from build123d import *

# Parameters (mm, degrees)
SKETCH_1_R       = 2.45
EXTRUDE_2_DEPTH  = 2
SKETCH_1_5_R     = 2.45
EXTRUDE_3_DEPTH  = 2
SKETCH_8_R       = 2.45
EXTRUDE_5_DEPTH  = 3
SKETCH_10_R      = 2.529452546
EXTRUDE_6_DEPTH  = 2
SKETCH_11_W      = 2.5
SKETCH_11_H      = 4.5
EXTRUDE_7_DEPTH  = 2
SKETCH_1_7_W     = 10
SKETCH_1_7_H     = 1
EXTRUDE_8_DEPTH  = 23
SKETCH_13_W      = 10
SKETCH_13_H      = 1
EXTRUDE_9_DEPTH  = 2
SKETCH_21_R      = 2.45
EXTRUDE_10_DEPTH = 5


with BuildPart() as part:
    # Sketch 1 → Extrude 2 (new body)
    with BuildSketch(Plane.XY):
        with BuildLine():
            Line((-52.360741066, -3.31033927), (-60.460741066, -3.31033927))
            Line((-60.460741066, -3.31033927), (-60.460741066, -7.81033927))
            Line((-60.460741066, -7.81033927), (-56.860741066, -7.81033927))
            ThreePointArc((-56.860741066, -7.81033927), (-49.178760551, -10.992319786), (-52.360741066, -3.31033927))
        make_face()
        with Locations((-52.360741066, -7.81033927)):
            Circle(SKETCH_1_R, mode=Mode.SUBTRACT)
    extrude(amount=-EXTRUDE_2_DEPTH)



with BuildPart() as body_2:
    # Sketch 1_5 → Extrude 3 (new body)
    with BuildSketch(Plane.XY):
        with BuildLine():
            Line((-78.460741066, -12.31033927), (-70.458584645, -12.31033927))
            Line((-70.458584645, -12.31033927), (-70.458584645, -13.81033927))
            Line((-70.458584645, -13.81033927), (-60.458584645, -13.81033927))
            Line((-60.458584645, -13.81033927), (-60.460741066, -12.31033927))
            Line((-60.460741066, -12.31033927), (-60.460741066, -7.81033927))
            Line((-60.460741066, -7.81033927), (-60.460741066, -3.31033927))
            Line((-60.460741066, -3.31033927), (-78.460741066, -3.31033927))
            ThreePointArc((-78.460741066, -3.31033927), (-82.960741066, -7.81033927), (-78.460741066, -12.31033927))
        make_face()
        with Locations((-78.460741066, -7.81033927)):
            Circle(SKETCH_1_5_R, mode=Mode.SUBTRACT)
    extrude(amount=EXTRUDE_3_DEPTH)


with BuildPart() as body_3:
    # Sketch 8 → Extrude 5 (new body)
    with BuildSketch(Plane.XY):
        with Locations((-52.360741066, -7.81033927)):
            Circle(SKETCH_8_R)
    extrude(amount=EXTRUDE_5_DEPTH)


with BuildPart() as part_1:
    add(part.part)

    add(body_3.part)  # Extrude 6 merges body 3
    # Sketch 10 → Extrude 6 (add)
    with BuildSketch(Plane.XY):
        with Locations((-52.43882399, -7.795650359)):
            Circle(SKETCH_10_R)
    extrude(amount=-EXTRUDE_6_DEPTH)


    add(body_2.part)  # Extrude 7 merges body 2
    # Sketch 11 → Extrude 7 (add)
    with BuildSketch(Plane(origin=(0, 0, 0), x_dir=(-1, 0, 0), z_dir=(0, 0, -1))):
        with Locations((61.710741066, -5.56033927)):
            Rectangle(SKETCH_11_W, SKETCH_11_H)
    extrude(amount=EXTRUDE_7_DEPTH)



with BuildPart() as body_2_2:
    # Sketch 1_7 → Extrude 8 (new body)
    with BuildSketch(Plane.XY):
        with Locations((-65.458584645, -14.31033927)):
            Rectangle(SKETCH_1_7_W, SKETCH_1_7_H)
    extrude(amount=-EXTRUDE_8_DEPTH)


with BuildPart() as part_2:
    add(part_1.part)

    add(body_2_2.part)  # Extrude 9 merges body 2 2
    # Sketch 13 → Extrude 9 (add)
    with BuildSketch(Plane.XY):
        with Locations((-65.458584645, -14.31033927)):
            Rectangle(SKETCH_13_W, SKETCH_13_H)
    extrude(amount=EXTRUDE_9_DEPTH)

    # Sketch 21 → Extrude 10 (add)
    with BuildSketch(Plane(origin=(0, 0, 0), x_dir=(-1, 0, 0), z_dir=(0, 0, -1))):
        with Locations((78.465233983, -7.801636169)):
            Circle(SKETCH_21_R)
    extrude(amount=-EXTRUDE_10_DEPTH)


solid = part_2.part
Geometry: final body of the model. Coordinates: model frame, mm. A direction names the side the tool comes from. Round coordinates to 2 decimals unless told otherwise and drop trailing zeros. Loops run counter-clockwise (first coordinate to the right, second up) from the corner with the lowest first, then second, coordinate; pieces in that order, holes last.
Q1. Section D-D on x = -51. Return loops of the section in (y, z), plus the area to 3 significant figures.
Q2. Section A-A on y = -8.25. Return loops of the section in (x, z), plus the area to 3 significant figures.
Q3. Pin query (flat end, axial travel): P1, Ø12, axis at x = -55, z = -7, coming from the +Y side; P2, Ø1, axis at x = -74, z = 1, coming from the -Y side; P3, Ø2.5, axis at x = -52, y = -6.5, coming from the +Z side; P4, Ø0.8, axis at y = -14, z = -10.5, coming from the -X side. Return the tip coordinate at first contact, or that it passes through.
Q4. Material intervals for L1, parallel to Z at x = -70, y = -14; L2, parallel to Y at x = -69.5, z = -2.25; L3, parallel to Z at x = -64, y = -5, sorted ascending.
Q5. Access query for faces 1 (the flat face through (-70.459, -14, -11)), 2 (the flat face through (-52, -8, 3)), 3 (the flat face through (-62.961, -6, -1)), 4 (the cylindrical face through (-82.96, -7.71, 0.99)), 5 (the flat face through (-54.2, -5.7, 0)). Directions: +Z, -Z, +X, -X, +Y, -Y. A direction counts if a zero-diameter tool reaches every point of the face in a straight line with its end or side. Return the directions, or none.
Q6. Section C-C on y = -11.5. Return loops of the section in (x, z).
Q7. Pull-direction query (Y, two-part tool) for faces 6 (the flat face through (-66, -14, -23)), 7 (the flat face through (-66, -14.81, -11)), 8 (the flat face through (-60, -7.81, -1)); classes: released by +Y, released by -Y, zero draft, split by the parting line, or undercut.
Q8. Section B-B on x = -79. Return loops of the section in (y, z).
Evaluation:
1. outline: (-12.1, -2) - (-3.52, -2) - (-3.52, 0) - (-5.77, 0) - (-5.77, 3) - (-9.85, 3) - (-9.85, 0) - (-12.1, 0) - close
1. area: 29.4 mm2
2. outline: (-82.94, 0) - (-76.06, 0) - (-76.06, 5) - (-80.87, 5) - (-80.87, 2) - (-82.94, 2) - close; (-76.05, 0) - (-60.46, 0) - (-60.46, 2) - (-76.05, 2) - close; (-56.84, -2) - (-47.88, -2) - (-47.88, 0) - (-49.95, 0) - (-49.95, 3) - (-54.77, 3) - (-54.77, 0) - (-56.84, 0) - close
2. area: 91.8 mm2
3. P1: stops at y = -3.31
3. P2: stops at y = -12.31
3. P3: stops at z = 3
3. P4: stops at x = -70.46
4. L1: z = -23 to 2
4. L2: y = -14.81 to -13.81
4. L3: z = 0 to 2
5. face 1: +Z, -Z, -X, -Y
5. face 2: +Z, +X, +Y, -Y
5. face 3: -Z, -X, +Y
5. face 4: +Z, -Z, -X
5. face 5: +Z
6. outline: (-81.04, 0) - (-60.46, 0) - (-60.46, 2) - (-81.04, 2) - close; (-54.94, -2) - (-49.78, -2) - (-49.78, 0) - (-54.94, 0) - close
7. face 6: zero draft
7. face 7: released by -Y
7. face 8: undercut
8. outline: (-12.28, 0) - (-10.2, 0) - (-10.2, 2) - (-12.28, 2) - close; (-10.19, 0) - (-3.34, 0) - (-3.34, 2) - (-5.41, 2) - (-5.41, 5) - (-10.19, 5) - close
